Can you work these out from the drawing? Everything is in mm from the part's minimum corner. A direction names the side the tool comes from. Round coordinates to 2 decimals unless told otherwise and drop trailing zeros. Write each loop counter-clockwise with the first axis right and the second up, starting at its lowest first coordinate (ties: lowest second). Pieces come first, ordered by that corner, then holes. Notation, with made-up numbers: (19, 58.5) -> (60, 58.5) arc R25 cw to (60, 86.5) -> close; hole circle Ø6 at (86, -13.75). An arc over 180 degrees is marked (long way). Answer as CSV lines item,"result".
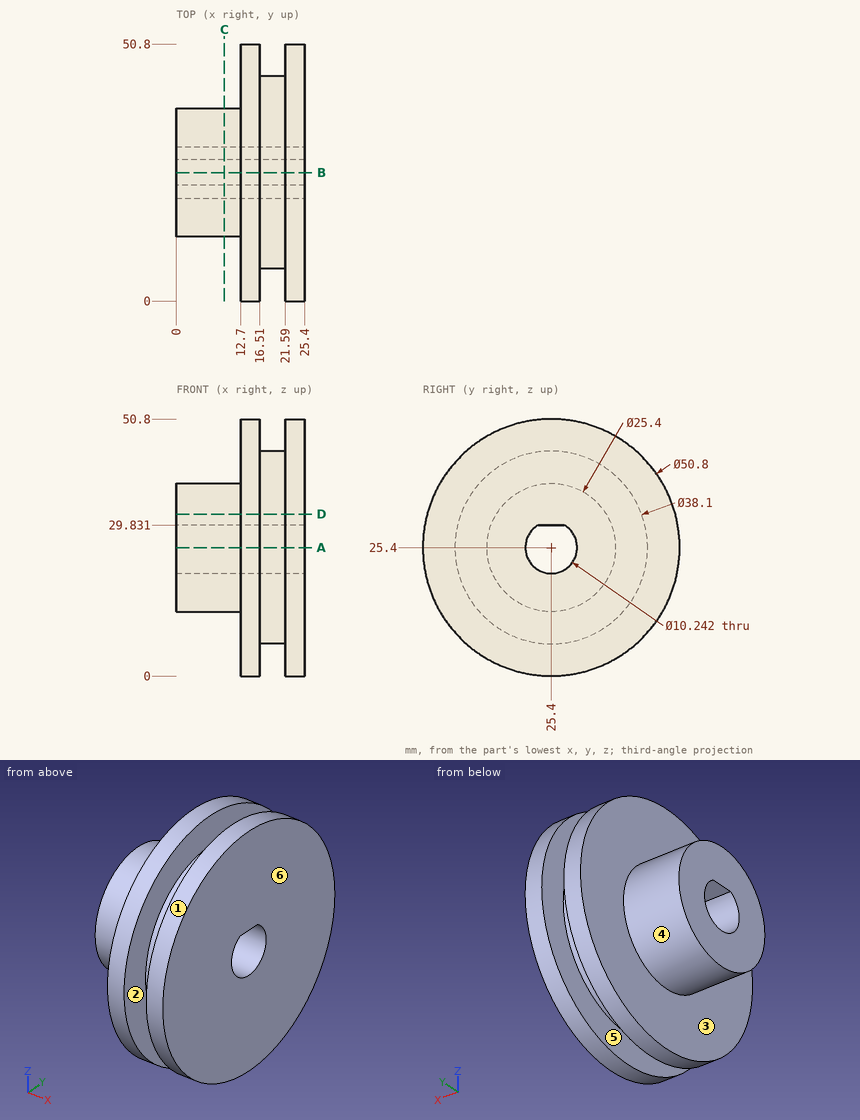
Item 1: Suppose I cut it at D-D, the plane z = 32. List the corners of the cut face in (x, y) for me, then the cut area to 3 significant figures.
Results found:
outline,"(0, 14.55) -> (12.7, 14.55) -> (12.7, 0.87) -> (16.51, 0.87) -> (16.51, 7.53) -> (21.59, 7.53) -> (21.59, 0.87) -> (25.4, 0.87) -> (25.4, 49.93) -> (21.59, 49.93) -> (21.59, 43.27) -> (16.51, 43.27) -> (16.51, 49.93) -> (12.7, 49.93) -> (12.7, 36.25) -> (0, 36.25) -> close"
area,"831 mm²"
Item 2: If we mould it in two halves opening along X, with no side actions, what happens to the marked faces 4, 5 and 6? For each: pulls with the +X half, pulls with the -X half, needs draft (parallel to the pull), parting line crosses it, or undercut.
Results found:
face 4,"needs draft"
face 5,"undercut"
face 6,"pulls with the +X half"
Item 3: Will these pins go through, and if not, where does the flat tip stop? pin 1 (1.5 mm diameter, centred on x = 20.5, y = 31, fed in from -Z); pin 2 (4 mm diameter, centred on x = 10.5, z = 27, fed in from +Y); pin 3 (8 mm diameter, centred on x = 5.5, y = 16, fed in from +Z).
Results found:
pin 1,"stops at z = 6.98"
pin 2,"stops at y = 38.1"
pin 3,"stops at z = 36.89"
Item 4: Suppose I cut it at C-C, the plane x = 9.5. List the corners of the cut face in (y, z) for me.
Results found:
outline,"circle Ø25.4 at (25.4, 25.4); hole (22.83, 29.83) arc R5.12 ccw (long way) to (27.97, 29.83) -> close"
Item 5: I need wall thicknesses on L1, parallel to X at y = 13.5, z = 3; L2, parallel to Z at x = 8.75, y = 25.4; L3, parallel to Z at x = 13.25, y = 25.4. Which ranges of each line are inside material? Lowest first, please.
Results found:
L1,"x = 12.7 to 16.51, 21.59 to 25.4"
L2,"z = 12.7 to 20.28, 29.83 to 38.1"
L3,"z = 0 to 20.28, 29.83 to 50.8"
Item 6: Suppose I cut it at B-B, the plane y = 25.4. List the corners of the cut face in (x, z) for me.
Results found:
outline,"(0, 12.7) -> (12.7, 12.7) -> (12.7, 0) -> (16.51, 0) -> (16.51, 6.35) -> (21.59, 6.35) -> (21.59, 0) -> (25.4, 0) -> (25.4, 20.28) -> (0, 20.28) -> close; (0, 29.83) -> (25.4, 29.83) -> (25.4, 50.8) -> (21.59, 50.8) -> (21.59, 44.45) -> (16.51, 44.45) -> (16.51, 50.8) -> (12.7, 50.8) -> (12.7, 38.1) -> (0, 38.1) -> close"
Item 7: Suppose I cut it at A-A, the plane z = 25.4. List the corners of the cut face in (x, y) for me, then the cut area to 3 significant figures.
Results found:
outline,"(0, 12.7) -> (12.7, 12.7) -> (12.7, 0) -> (16.51, 0) -> (16.51, 6.35) -> (21.59, 6.35) -> (21.59, 0) -> (25.4, 0) -> (25.4, 20.28) -> (0, 20.28) -> close; (0, 30.52) -> (25.4, 30.52) -> (25.4, 50.8) -> (21.59, 50.8) -> (21.59, 44.45) -> (16.51, 44.45) -> (16.51, 50.8) -> (12.7, 50.8) -> (12.7, 38.1) -> (0, 38.1) -> close"
area,"643 mm²"
Item 8: For the marked faces 1, 2 and 3, which set-ups out of +Z, -Z, +X, -X, +Y, -Y let a thin tool reach every point of the face, with its end or its side?
Results found:
face 1,"+X, -X"
face 2,"none"
face 3,"-X"
